Study the drawing (mm; zero at the part's minimum x, y, z) and answer. Give positions to 0.01 mm unless a question says otherwise; leave off trailing zeros. Order: outer loops, then holes, each group sorted by start corner. A loop starts at its lowest first (then second) coordinate and runs counter-clockwise, first axis right, second up. Notation, with made-up numbers: (24.25, -22.75) - (55.25, -22.75) arc R28 ccw to (55.25, 16.25) - close; hole circle Ø8 at (7, 21). An arc over 180 degrees is marked (long way). Return JSON: item names as keys, results as strings.
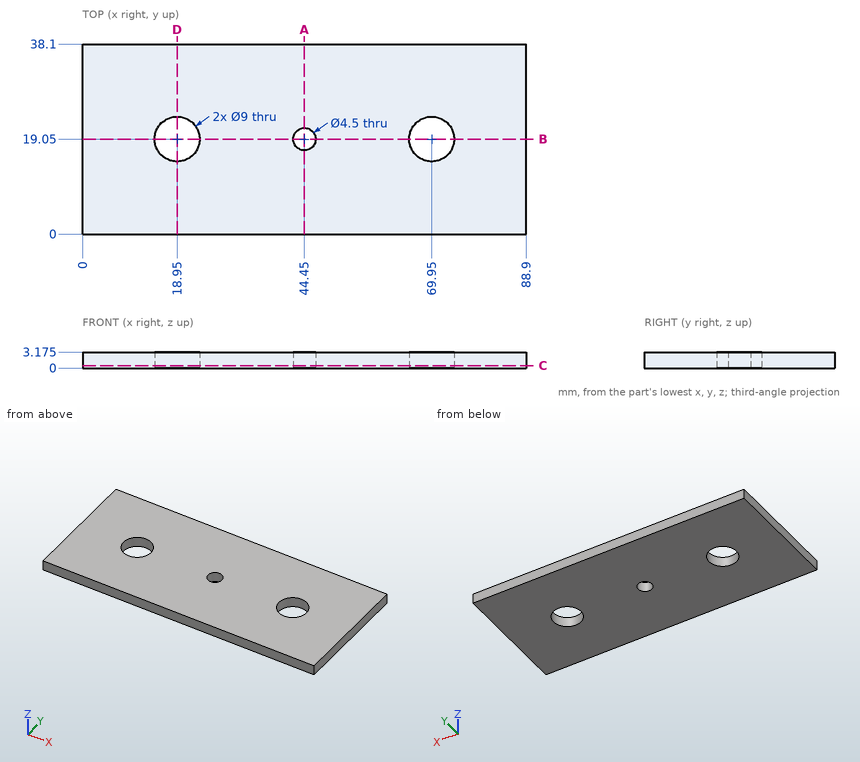
Q1. A cutting plane is placed at C-C (z = 0.5). Write down the section's boundary in (x, y), and give its area (3 significant figures).
Values:
{"outline": "(0, 0) - (88.9, 0) - (88.9, 38.1) - (0, 38.1) - close; hole circle Ø9 at (18.95, 19.05); hole circle Ø4.5 at (44.45, 19.05); hole circle Ø9 at (69.95, 19.05)", "area": "3,240 mm²"}
Q2. A cutting plane is placed at B-B (y = 19.05). Write down the section's boundary in (x, z) (3 decimals).
Values:
{"outline": "(0, 0) - (14.45, 0) - (14.45, 3.175) - (0, 3.175) - close; (23.45, 0) - (42.2, 0) - (42.2, 3.175) - (23.45, 3.175) - close; (46.7, 0) - (65.45, 0) - (65.45, 3.175) - (46.7, 3.175) - close; (74.45, 0) - (88.9, 0) - (88.9, 3.175) - (74.45, 3.175) - close"}
Q3. Given pin 1 (6 mm diameter, centred on x = 45.5, y = 20, fed in from +Z) (3 decimals), flat-ended and moving along its own axis, determine where the tip first touches the part or whether it passes through.
Values:
{"pin 1": "stops at z = 3.175"}
Q4. A cutting plane is placed at A-A (x = 44.45). Write down the section's boundary in (y, z) (3 decimals), and give its area (3 significant figures).
Values:
{"outline": "(0, 0) - (16.8, 0) - (16.8, 3.175) - (0, 3.175) - close; (21.3, 0) - (38.1, 0) - (38.1, 3.175) - (21.3, 3.175) - close", "area": "107 mm²"}
Q5. A cutting plane is placed at D-D (x = 18.95). Write down the section's boundary in (y, z) (3 decimals), and give its area (3 significant figures).
Values:
{"outline": "(0, 0) - (14.55, 0) - (14.55, 3.175) - (0, 3.175) - close; (23.55, 0) - (38.1, 0) - (38.1, 3.175) - (23.55, 3.175) - close", "area": "92.4 mm²"}
Q6. Consider L1, parallel to X at y = 15, z = 2.15; L2, parallel to Y at x = 18.95, z = 2.1; L3, parallel to X at y = 22.5, z = 2.7. Determine where each line is inside the solid, lowest interval first.
Values:
{"L1": "x = 0 to 16.99, 20.91 to 67.99, 71.91 to 88.9", "L2": "y = 0 to 14.55, 23.55 to 38.1", "L3": "x = 0 to 16.06, 21.84 to 67.06, 72.84 to 88.9"}
